Check sheet for the modelled part. Datum: model origin and axes. Units: mm. Face numbers are marked on the shaded views. A direction names the side the tool comes from. Coordinates: 2 decimals unless noted, no trailing zeros. Loops run counter-clockwise (first coordinate to the right, second up) from the corner with the lowest first, then second, coordinate; pieces in that order, holes last. Notation, with made-up numbers: M -1,62 L 33,62 A19 ccw 33,86 Z; hole C 60.25,-5 d5. An arc over 180 degrees is marked long. Use CSV: the item, a comma, the result in double quotes. Start each with the question number.
(1) Section check A-A on x = 0. Record the cut outline in (y, z).
(2) Section check D-D on x = -6. Record the cut outline in (y, z).
(3) Scan lines: line 1 (Y direction, x = -13, z = 0.5); line 2 (Z direction, x = -3.5, y = -5.25); line 3 (Z direction, x = -4.5, y = -3.25). Record each from-to range of solid material in increasing order.
(4) Section check B-B on z = 13.5. Record the cut outline in (x, y).
(5) Draft check along Z on the marked faces 1, 2 and 3. Enter one of: pulls with the +Z half, pulls with the -Z half, needs draft (parallel to the pull), parting line crosses it, or undercut.
(6) Go/stop test with flat-tipped pins: pin 1 Ø3 at (y, z) = (-2.5, 3) entering from +X; pin 2 Ø1 at (x, y) = (5.5, -1.5) entering from -Z; pin 3 Ø2.5 at (x, z) = (14.07, -0.04) entering from +Y. Record where each tip stops, or that it passes through.
(7) Section check C-C on y = -4. Record the cut outline in (x, z), and give its area (3 significant figures).
(8) Set-up check for the marked faces 4 and 5: record each of +Z, -Z, +X, -X, +Y, -Y from which the full face is reachable in a straight line by a thin tool's end or side.
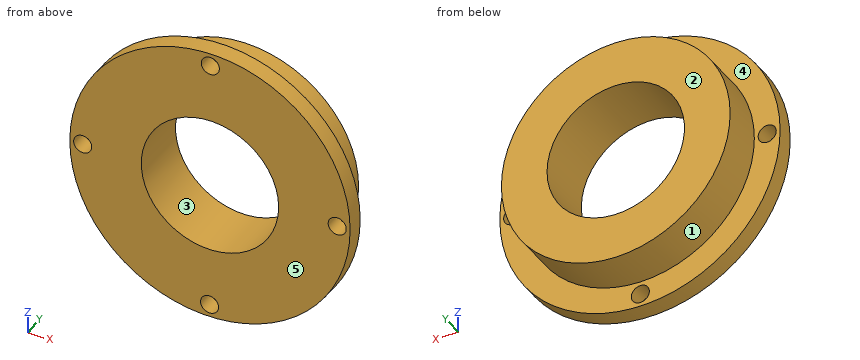
from build123d import *

# Parameters (mm, degrees)
F0_R     = 12.65
F1_DEPTH = 4.8
F2_R     = 15.5
F2_R_2   = 12.65
F3_DEPTH = 2
F4_R     = 1
F5_DEPTH = 2
F6_R     = 7.6
F7_DEPTH = 7


# Not quite as in the source:
# - a feature names something its author has since deleted; it is built from what else it names


with BuildPart() as f1:
    # F0 (on Front) → F1 (new body)
    with BuildSketch(Plane.XZ):
        Circle(F0_R)
    extrude(amount=F1_DEPTH)

    # F2 (on face) → F3 (join)
    with BuildSketch(Plane.XZ.offset(4.8)):
        Circle(F2_R)
        Circle(F2_R_2, mode=Mode.SUBTRACT)
        Circle(F2_R_2)
    extrude(amount=F3_DEPTH)

    # F4 (on face) → F5 (cut)
    with BuildSketch(Plane(origin=(0, -4.8, 0), x_dir=(-1, 0, 0), z_dir=(0, 1, 0))):
        with Locations((-0.0435703545, 14.074932562)):
            Circle(F4_R)
        with Locations((-14.074932562, -0.0435703545)):
            Circle(F4_R)
        with Locations((0.0435703545, -14.074932562)):
            Circle(F4_R)
        with Locations((14.074932562, 0.0435703545)):
            Circle(F4_R)
    extrude(amount=-F5_DEPTH, mode=Mode.SUBTRACT)

    # F6 (on face) → F7 (cut)
    with BuildSketch(Plane.XZ.offset(6.8)):
        Circle(F6_R)
    extrude(amount=-F7_DEPTH, mode=Mode.SUBTRACT)


solid = f1.part
Outcome:
1,outline,"M -6.8,-15.5 L -4.8,-15.5 L -4.8,-15.07 L -6.8,-15.07 Z; M -6.8,-13.08 L -4.8,-13.08 L -4.8,-12.65 L 0,-12.65 L 0,-7.6 L -6.8,-7.6 Z; M -6.8,7.6 L 0,7.6 L 0,12.65 L -4.8,12.65 L -4.8,13.08 L -6.8,13.08 Z; M -6.8,15.07 L -4.8,15.07 L -4.8,15.5 L -6.8,15.5 Z"
2,outline,"M -6.8,-14.29 L -4.8,-14.29 L -4.8,-11.14 L 0,-11.14 L 0,-4.66 L -6.8,-4.66 Z; M -6.8,4.66 L 0,4.66 L 0,11.14 L -4.8,11.14 L -4.8,14.29 L -6.8,14.29 Z"
3,line 1,"y = -6.8 to -4.8"
3,line 2,"z = -15.1 to -6.75, 6.75 to 15.1"
3,line 3,"z = -11.82 to -6.12, 6.12 to 11.82"
4,outline,"M -7.62,-6.8 L -0.77,-6.8 L -0.77,-4.8 L -7.62,-4.8 Z; M 0.86,-6.8 L 7.62,-6.8 L 7.62,-4.8 L 0.86,-4.8 Z"
5,face 1,"parting line crosses it"
5,face 2,"needs draft"
5,face 3,"undercut"
6,pin 1,"stops at x = 12.56"
6,pin 2,"stops at z = -11.62"
6,pin 3,"stops at y = -4.8"
7,outline,"C 0,0 d25.3; hole C 0,0 d15.2"
7,area,"321 mm²"
8,face 4,"+Y"
8,face 5,"+Z, -Z, +X, -X, -Y"
